Could you check a few things on this model? Use its own coordinates, in mm. A direction names the side the tool comes from. Coordinates: 2 decimals unless noted, no trailing zeros. Order: outer loops, then holes, each group sorted by start corner. A loop starts at its lowest first (then second) coordinate and runs counter-clockwise, first axis right, second up. Notation, with made-up numbers: (-20.5, -5) - (-6.5, -5) arc R24 cw to (-6.5, 30) - close; hole circle Ø1 at (-30.75, -8.5). An arc over 180 degrees is marked (long way). One line per item, written item: value.
from build123d import *

# Parameters (mm, degrees)
SKETCH2_W                    = 75
SKETCH2_H                    = 100
BOSS_EXTRUDE1_DEPTH          = 10
SKETCH5_R                    = 25
BOSS_EXTRUDE4_DEPTH          = 10
F_5_0_5_DIAMETER_HOLE1_D     = 5
F_12_0_12_DIAMETER_HOLE1_D   = 12
CUT_EXTRUDE1_DEPTH           = 6
FILLET1_R                    = 10
F_3_0_3_DIAMETER_HOLE1_D     = 3
F_3_0_3_DIAMETER_HOLE1_DEPTH = 10
F_3_0_3_DIAMETER_HOLE1_TIP   = 0.901290929
SKETCH18_W                   = 17
SKETCH18_H                   = 8
BOSS_EXTRUDE5_DEPTH          = 3
FILLET2_R                    = 4


with BuildPart() as part:
    # Sketch2 → Boss-Extrude1 (new body)
    with BuildSketch(Plane.XY):
        with Locations((37.5, 50)):
            Rectangle(SKETCH2_W, SKETCH2_H)
    extrude(amount=BOSS_EXTRUDE1_DEPTH)

    # Sketch5 → Boss-Extrude4 (add)
    with BuildSketch(Plane.XY.offset(10)):
        with Locations((40, 40)):
            Circle(SKETCH5_R)
    extrude(amount=BOSS_EXTRUDE4_DEPTH)

    # Ø5.0 (5) Diameter Hole1 (through all)
    with Locations(Plane.XY.offset(20)):
        with Locations((31.161165235, 48.838834765), (48.838834765, 48.838834765)):
            Hole(F_5_0_5_DIAMETER_HOLE1_D / 2)

    # Ø12.0 (12) Diameter Hole1 (through all)
    with Locations(Plane.XY.offset(20)):
        with Locations((40, 35)):
            Hole(F_12_0_12_DIAMETER_HOLE1_D / 2)

    # Sketch12 → Cut-Extrude1 (cut)
    with BuildSketch(Plane.XY.offset(10)):
        with BuildLine():
            Line((15, 89), (65, 89))
            ThreePointArc((65, 89), (69, 85), (65, 81))
            Line((65, 81), (15, 81))
            ThreePointArc((15, 81), (11, 85), (15, 89))
        make_face()
    extrude(amount=-CUT_EXTRUDE1_DEPTH, mode=Mode.SUBTRACT)

    # Fillet1
    fillet1_edges = [part.edges().sort_by_distance(p)[0] for p in [
        (0, 100, 5),
        (75, 100, 5),
        (75, 0, 5),
        (0, 0, 5),
    ]]
    fillet(fillet1_edges, radius=FILLET1_R)

    # Ø3.0 (3) Diameter Hole1
    with Locations(Plane.XY.offset(10)):
        with Locations((15, 73), (37.5, 73), (60, 73)):
            Hole(F_3_0_3_DIAMETER_HOLE1_D / 2, depth=F_3_0_3_DIAMETER_HOLE1_DEPTH)
            with Locations((0, 0, -(F_3_0_3_DIAMETER_HOLE1_DEPTH + F_3_0_3_DIAMETER_HOLE1_TIP / 2))):  # 118° drill point
                Cone(0, F_3_0_3_DIAMETER_HOLE1_D / 2, F_3_0_3_DIAMETER_HOLE1_TIP, mode=Mode.SUBTRACT)

    # Sketch18 → Boss-Extrude5 (add)
    with BuildSketch(Plane.XY.offset(4)):
        with Locations((43.5, 85)):
            Rectangle(SKETCH18_W, SKETCH18_H)
    extrude(amount=BOSS_EXTRUDE5_DEPTH)

    # Fillet2
    fillet2_edges = [part.edges().sort_by_distance(p)[0] for p in [
        (52, 81, 5.5),
        (52, 89, 5.5),
        (35, 81, 5.5),
        (35, 89, 5.5),
    ]]
    fillet(fillet2_edges, radius=FILLET2_R - 0.0001)  # a hair under: the kernel refuses the full size


solid = part.part
Item 1: I want a section at D-D on x = 47.5. Please give me the cut outline in (y, z).
Conclusion:
outline: (0, 0) - (46.73, 0) - (46.73, 20) - (16.15, 20) - (16.15, 10) - (0, 10) - close; (50.95, 0) - (100, 0) - (100, 10) - (89, 10) - (89, 7) - (81, 7) - (81, 10) - (63.85, 10) - (63.85, 20) - (50.95, 20) - close
Item 2: If I drill on probe 1 along Y at (x, z) = (15, 6); probe 2 along X at (y, z) = (73, 2.25); probe 3 along X at (y, z) = (48, 13.25), over which ranges is the centre line in solid material (lowest first)?
Conclusion:
probe 1: 0 to 71.5, 74.5 to 81, 89 to 100
probe 2: 0 to 13.5, 16.5 to 36, 39 to 58.5, 61.5 to 75
probe 3: 16.31 to 28.81, 33.52 to 46.48, 51.19 to 63.69
Item 3: I'm going to push flat-ended pins straight in: pin 1 Ø8 at (x, y) = (28, 21.5) entering from -Z; pin 2 Ø3.5 at (x, y) = (15, 73) entering from +Z; pin 3 Ø4 at (x, y) = (21, 85.5) entering from +Z; pin 4 Ø8 at (x, z) = (54, 16) entering from -Y. Where does each tip first touch, or does it pass through?
Conclusion:
pin 1: z = 0
pin 2: z = 10
pin 3: z = 4
pin 4: y = 17.09
Item 4: I want a section at B-B on x = 37.5. Please give me the cut outline in (y, z), then the cut area to 3 significant figures.
Conclusion:
outline: (0, 0) - (29.55, 0) - (29.55, 20) - (15.13, 20) - (15.13, 10) - (0, 10) - close; (40.45, 0) - (71.5, 0) - (71.5, 10) - (64.87, 10) - (64.87, 20) - (40.45, 20) - close; (74.5, 0) - (100, 0) - (100, 10) - (89, 10) - (89, 7) - (81, 7) - (81, 10) - (74.5, 10) - close
area: 1,230 mm²
Item 5: I want a section at A-A on y = 73. Please give me the cut outline in (x, z).
Conclusion:
outline: (0, 0) - (13.5, 0) - (13.5, 10) - (0, 10) - close; (16.5, 0) - (36, 0) - (36, 10) - (16.5, 10) - close; (39, 0) - (58.5, 0) - (58.5, 10) - (39, 10) - close; (61.5, 0) - (75, 0) - (75, 10) - (61.5, 10) - close
Item 6: Thinking about a two-plate mould opening in X: for faces 1 (the face through (40, 89, 8)), 2 (the face through (45, 40, 20)), 3 (the face through (0, 49, 5)), which applies, pulls with the +X half, pulls with the -X half, needs draft (parallel to the pull), parting line crosses it, or undercut?
Conclusion:
face 1: undercut
face 2: needs draft
face 3: pulls with the -X half
Item 7: I want a section at C-C on y = 38.5. Please give me the cut outline in (x, z), then the cut area to 3 significant figures.
Conclusion:
outline: (0, 0) - (35.13, 0) - (35.13, 20) - (15.05, 20) - (15.05, 10) - (0, 10) - close; (44.87, 0) - (75, 0) - (75, 10) - (64.95, 10) - (64.95, 20) - (44.87, 20) - close
area: 1,050 mm²
Item 8: For faces 4 (the face through (33.797, 87.859, 5.521)), 5 (the face through (37, 100, 5)), which set-ups out of +Z, -Z, +X, -X, +Y, -Y let a thin tool reach every point of the face, with its end or its side?
Conclusion:
face 4: +Z
face 5: +Z, -Z, +X, -X, +Y
